Autodesk Inventor part; units mm, degrees
ref_plane "YZ Plane" through (0, 0, 0) normal (1, 0, 0) x (0, 1, 0)
ref_plane "XZ Plane" through (0, 0, 0) normal (0, 1, 0) x (-1, 0, 0)
ref_plane "XY Plane" through (0, 0, 0) normal (0, 0, 1) x (1, 0, 0)
sketch "Sketch1" plane through (0, 0, 0) normal (0, 1, 0) x (-1, 0, 0)
  line L0 (16, -28.5) -> (-16, -28.5)
  line L1 (-16, -28.5) -> (-16, 28.5)
  line L2 (-16, 28.5) -> (16, 28.5)
  line L3 (16, 28.5) -> (16, -28.5)
  line L4 (16, -28.5) -> (-16, 28.5) construction
  line L5 (-16, -28.5) -> (16, 28.5) construction
  point P0 (0, 0)
  dimension "d0" = 32
  dimension "d1" = 57
extrude "Extrusion1" add sketch "Sketch1" along normal blind 1
sketch "Sketch2" plane through (0, 1, 0) normal (0, 1, 0) x (1, 0, 0)
  line L0 (-9.5, -27.5) -> (9.5, -27.5)
  line L1 (15.5, -25.5) -> (15.5, 25.5)
  line L2 (9.5, 27.5) -> (-9.5, 27.5)
  line L3 (-15.5, 25.5) -> (-15.5, -25.5)
  line L4 (-15.5, -27.5) -> (15.5, 27.5) construction
  line L5 (15.5, -27.5) -> (-15.5, 27.5) construction
  line L6 (13.5, -25.5) -> (13.5, 25.5)
  line L7 (-13.5, 25.5) -> (-13.5, -25.5)
  line L8 (-16, -28.5) -> (16, -28.5)
  line L9 (-9.5, -28.4306) -> (-9.5, -25.5)
  line L10 (9.5, 25.5) -> (9.5, 27.5)
  line L11 (-9.5, -16.8548) -> (-9.5, 16.8548)
  line L12 (-9.5, 25.5) -> (-9.5, 28.5928)
  line L13 (9.5, -28.5) -> (9.5, -25.5)
  line L14 (9.5, -16.8548) -> (9.5, 16.8548)
  line L15 (13.5, -25.5) -> (15.5, -25.5)
  line L16 (15.5, 25.5) -> (13.5, 25.5)
  line L17 (9.5, 25.5) -> (-9.5, 25.5)
  line L18 (-13.5, 25.5) -> (-15.5, 25.5)
  line L19 (-15.5, -25.5) -> (-13.5, -25.5)
  line L20 (-9.5, -25.5) -> (9.5, -25.5)
  point P0 (0, 0)
  dimension "d4" = 31
  dimension "d5" = 55
  dimension "d6" = 2
extrude "Extrusion2" add sketch "Sketch2" along normal blind 4
sketch "Sketch3" plane through (15.5, 1, 25.5) normal (1, 0, 0) x (0, 0, -1)
  circle A0 centre (25.5, 6.5) radius 5
  line L0 (-3, 0) -> (54, 0)
  point P0 (25.5, -1)
  dimension "d11" = 10
  dimension "d12" = 6.5
extrude "Extrusion3" cut sketch "Sketch3" against normal through all
sketch "Sketch4" plane through (0, 0, 0) normal (0, -1, 0) x (1, 0, 0)
  line L0 (7.5, -7.5) -> (-7.5, -7.5)
  line L1 (-7.5, -7.5) -> (-7.5, 7.5)
  line L2 (-7.5, 7.5) -> (7.5, 7.5)
  line L3 (7.5, 7.5) -> (7.5, -7.5)
  line L4 (7.5, -7.5) -> (-7.5, 7.5) construction
  line L5 (-7.5, -7.5) -> (7.5, 7.5) construction
  point P0 (0, 0)
  dimension "d15" = 15
  dimension "d16" = 15
extrude "Extrusion4" cut sketch "Sketch4" against normal through all
sketch "Sketch5" plane through (0, 1, 0) normal (0, 1, 0) x (1, 0, 0)
  line L0 (7.5, 7.5) -> (7.5, -7.5)
  line L1 (7.5, -7.5) -> (-7.5, -7.5)
  line L2 (-7.5, -7.5) -> (-7.5, 7.5)
  line L3 (-7.5, 7.5) -> (7.5, 7.5)
  line L4 (-13.5, -25.5) -> (-15.5, -25.5)
  line L5 (-15.5, -25.5) -> (-15.5, 25.5)
  line L6 (-15.5, 25.5) -> (-13.5, 25.5)
  line L7 (-13.5, 25.5) -> (-13.5, -25.5)
  line L8 (9.5, -27.5) -> (-9.5, -27.5)
  line L9 (-9.5, -27.5) -> (-9.5, -25.5)
  line L10 (-9.5, -25.5) -> (9.5, -25.5)
  line L11 (9.5, -25.5) -> (9.5, -27.5)
  line L12 (9.5, 27.5) -> (9.5, 25.5)
  line L13 (9.5, 25.5) -> (-9.5, 25.5)
  line L14 (-9.5, 25.5) -> (-9.5, 27.5)
  line L15 (-9.5, 27.5) -> (9.5, 27.5)
  line L16 (13.5, 25.5) -> (15.5, 25.5)
  line L17 (15.5, 25.5) -> (15.5, -25.5)
  line L18 (15.5, -25.5) -> (13.5, -25.5)
  line L19 (13.5, -25.5) -> (13.5, 25.5)
  line L20 (16, 28.5) -> (-16, 28.5)
  line L21 (-16, 28.5) -> (-16, -28.5)
  line L22 (-16, -28.5) -> (16, -28.5)
  line L23 (16, -28.5) -> (16, 28.5)
  line L24 (-8.5, -8.5) -> (8.5, -8.5)
  line L25 (8.5, -8.5) -> (8.5, 8.5)
  line L26 (8.5, 8.5) -> (-8.5, 8.5)
  line L27 (-8.5, 8.5) -> (-8.5, -8.5)
  point P0 (0, 0)
  dimension "d19" = 1
extrude "Extrusion5" add sketch "Sketch5" along normal blind 1 contours L27 L26 L25 L24
properties part number "hull_cover"
Read the model definition and answer for the solid it produces. Units are mm, in the model's axes. A direction names the side the tool comes from. Give positions to 0.01 mm unless a question says otherwise; leave off trailing zeros. Order: outer loops, then holes, each group sorted by start corner. A loop starts at its lowest first (then second) coordinate and runs counter-clockwise, first axis right, second up.
(1) For a pull along X with two mould halves and no side action, classify faces 6 (the flat face through (16, 0.5, -0.4)), 7 (the flat face through (0, 3, 25.5)), 8 (the flat face through (11, 0, 0)), 9 (the flat face through (13.5, 2, 0)) as released by +X, released by -X, zero draft, split by the parting line, or undercut.
(2) Given pin 1 (0.8 mm diameter, centred on y = 1.5, z = -2, fed in from -X); pin 2 (1 mm diameter, centred on y = 3.5, z = -26.5, fed in from +X); pin 3 (3 mm diameter, centred on x = -3.5, y = 3.5, fed in from +Z), each flat-ended and moving along its own axis, determine where each tip first touches the part or whether it passes through.
(3) Find section C-C (z = 3.5). Give the vertices of the cut face in (x, y).
(4) Find section D-D (z = -15.5). Give the vertices of the cut face in (x, y).
(5) Find section B-B (y = 4). Give the vertices of the cut face in (x, z), plus the area to 3 significant figures.
(6) Find section A-A (x = 6). Give the vertices of the cut face in (y, z), plus the area to 3 significant figures.
(7) For faces 1 (the flat face through (9.5, 3, -26)), 2 (the flat face through (0, 3, -27.5)), 3 (the flat face through (0.1, 1.5, -8.5)), 4 (the flat face through (-14, 3, -25.5)), 5 (the flat face through (-7.5, 1, 0)), determine the directions among +Z, -Z, +X, -X, +Y, -Y from which every point of the face is accessible in a straight line to the end or side of a thin tool.
(8) Straight lines are drawn through the part: L1, parallel to Z at x = 0, y = 1.95; L2, parallel to X at y = 2.25, z = -16.5; L3, parallel to Z at x = 6, y = 2.7. For each, find the intervals that lie inside material, in ascending order.
Result sheet:
1. face 6: released by +X
1. face 7: undercut
1. face 8: zero draft
1. face 9: undercut
2. pin 1: stops at x = -15.5
2. pin 2: stops at x = 9.5
2. pin 3: stops at z = 27.5
3. outline: (-16, 0) - (-7.5, 0) - (-7.5, 2) - (-8.5, 2) - (-8.5, 1) - (-13.5, 1) - (-13.5, 3.93) - (-15.5, 3.93) - (-15.5, 1) - (-16, 1) - close; (7.5, 0) - (16, 0) - (16, 1) - (15.5, 1) - (15.5, 3.93) - (13.5, 3.93) - (13.5, 1) - (8.5, 1) - (8.5, 2) - (7.5, 2) - close
4. outline: (-16, 0) - (16, 0) - (16, 1) - (15.5, 1) - (15.5, 5) - (13.5, 5) - (13.5, 1) - (-13.5, 1) - (-13.5, 5) - (-15.5, 5) - (-15.5, 1) - (-16, 1) - close
5. outline: (-15.5, -25.5) - (-13.5, -25.5) - (-13.5, -3.57) - (-15.5, -3.57) - close; (-15.5, 3.57) - (-13.5, 3.57) - (-13.5, 25.5) - (-15.5, 25.5) - close; (-9.5, -27.5) - (9.5, -27.5) - (9.5, -25.5) - (-9.5, -25.5) - close; (-9.5, 25.5) - (9.5, 25.5) - (9.5, 27.5) - (-9.5, 27.5) - close; (13.5, -25.5) - (15.5, -25.5) - (15.5, -3.57) - (13.5, -3.57) - close; (13.5, 3.57) - (15.5, 3.57) - (15.5, 25.5) - (13.5, 25.5) - close
5. area: 251 mm2
6. outline: (0, -28.5) - (1, -28.5) - (1, -27.5) - (5, -27.5) - (5, -25.5) - (1, -25.5) - (1, -8.5) - (2, -8.5) - (2, -7.5) - (0, -7.5) - close; (0, 7.5) - (2, 7.5) - (2, 8.5) - (1, 8.5) - (1, 25.5) - (5, 25.5) - (5, 27.5) - (1, 27.5) - (1, 28.5) - (0, 28.5) - close
6. area: 60.0 mm2
7. face 1: +Z, -Z, +X, +Y
7. face 2: -Z, +X, -X, +Y
7. face 3: +Y
7. face 4: -Z, -X, +Y
7. face 5: +Y, -Y
8. L1: z = -27.5 to -25.5, -8.5 to -7.5, 7.5 to 8.5, 25.5 to 27.5
8. L2: x = -15.5 to -13.5, 13.5 to 15.5
8. L3: z = -27.5 to -25.5, 25.5 to 27.5
